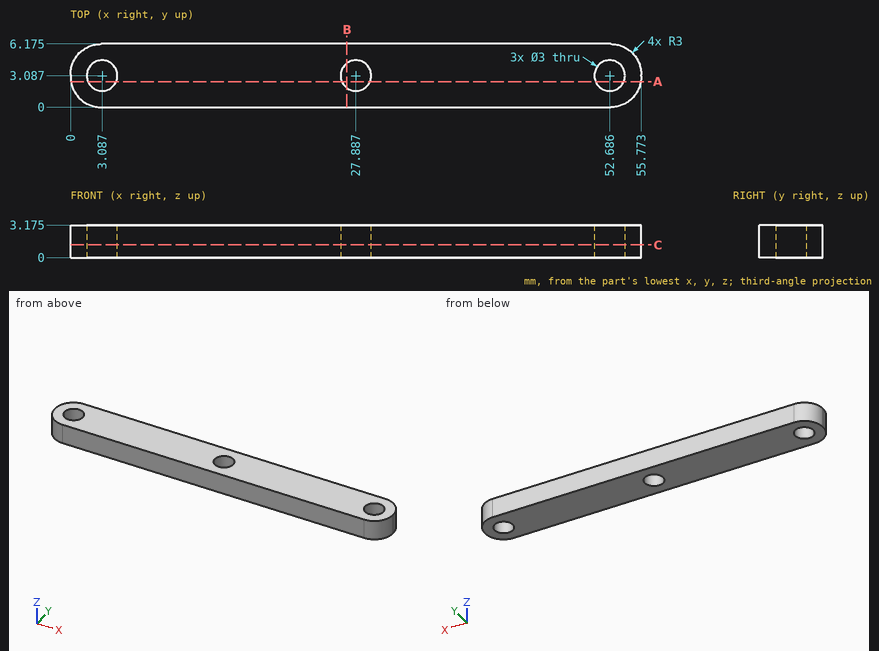
Source: three-view drawing plus pictorial views. Frame: mm from the lowest corner of the part. Round coordinates to 2 decimals unless told otherwise and drop trailing zeros. Loops run counter-clockwise (first coordinate to the right, second up) from the corner with the lowest first, then second, coordinate; pieces in that order, holes last.
1. Section query A-A on y = 2.5. Output: boundary loops of the cut face in (x, z) (1 decimal).
2. Section query C-C on z = 1.25. Give the number of separate pieces and of enclosed holes in the cut face.
3. Contact query for a flat-ended pin moving along its axis: pin 1 (2.5 mm diameter, centred on x = 27.89, y = 3.09, fed in from -Z). Output: stop coordinate, or through.
4. Ray query, L1, parallel to X at y = 3.25, z = 1.15 (1 decimal); L2, parallel to X at y = 2.25, z = 1.2 (1 decimal); L3, parallel to Y at x = 52.5, z = 2.8 (1 decimal). Return the intervals inside material, ascending.
5. Section query B-B on x = 27. Output: boundary loops of the cut face in (y, z) (1 decimal), and give its area (3 significant figures).
Answers below:
1. outline: (0, 0) - (1.7, 0) - (1.7, 3.2) - (0, 3.2) - close; (4.5, 0) - (26.5, 0) - (26.5, 3.2) - (4.5, 3.2) - close; (29.3, 0) - (51.3, 0) - (51.3, 3.2) - (29.3, 3.2) - close; (54.1, 0) - (55.7, 0) - (55.7, 3.2) - (54.1, 3.2) - close
2. separate pieces: 1
2. enclosed holes: 3
3. pin 1: passes through
4. L1: x = 0 to 1.6, 4.6 to 26.4, 29.4 to 51.2, 54.2 to 55.8
4. L2: x = 0.1 to 1.8, 4.3 to 26.6, 29.1 to 51.4, 53.9 to 55.7
4. L3: y = 0 to 1.6, 4.6 to 6.2
5. outline: (0, 0) - (1.9, 0) - (1.9, 3.2) - (0, 3.2) - close; (4.3, 0) - (6.2, 0) - (6.2, 3.2) - (4.3, 3.2) - close
5. area: 11.9 mm2
